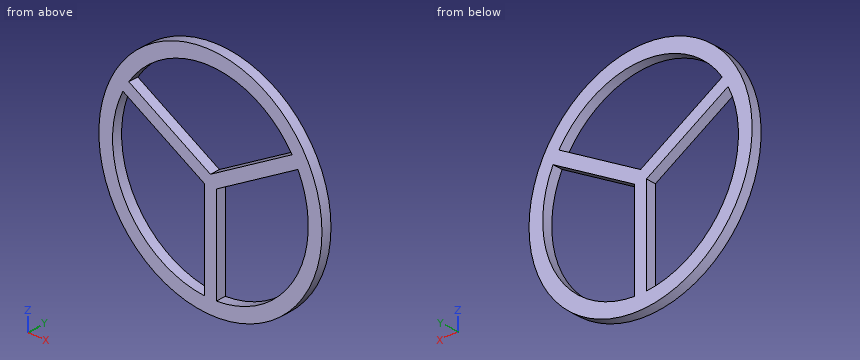
```python
from build123d import *

# Parameters (mm, degrees)
SKETCH1_R           = 28.5
SKETCH1_R_2         = 25
BOSS_EXTRUDE1_DEPTH = 2.5
BOSS_EXTRUDE2_DEPTH = 2.5


with BuildPart() as part:
    # Sketch1 → Boss-Extrude1 (new body)
    with BuildSketch(Plane(origin=(0, 0, 0), x_dir=(1, 0, 0), z_dir=(0, 1, 0))):
        Circle(SKETCH1_R)
        Circle(SKETCH1_R_2, mode=Mode.SUBTRACT)
    extrude(amount=BOSS_EXTRUDE1_DEPTH)

    # Sketch2 → Boss-Extrude2 (add)
    with BuildSketch(Plane(origin=(0, 2.5, 0), x_dir=(1, 0, 0), z_dir=(0, 1, 0))):
        Polygon((-1.5, 0.866025404), (-22.400635095, -11.200961894), (-20.900635095, -13.799038106), (0, -1.732050808), (20.900635095, -13.799038106), (22.400635095, -11.200961894), (1.5, 0.866025404), (1.5, 25), (-1.5, 25), align=None)
    extrude(amount=-BOSS_EXTRUDE2_DEPTH)


solid = part.part
```
Work out the finished part from the listing and answer in its coordinate system (mm). Round coordinates to 2 decimals unless told otherwise and drop trailing zeros. Write each loop counter-clockwise with the first axis right and the second up, starting at its lowest first coordinate (ties: lowest second). Pieces come first, ordered by that corner, then holes. Notation, with made-up numbers: (26, 62) -> (49, 62) arc R10 ccw to (49, 77) -> close; hole circle Ø6 at (83.25, -6.75). An arc over 180 degrees is marked (long way). Write each question's results on one line, items separated by ' | '.
1) The part is cut by section A-A (y = 1.3). Write down the section's boundary in (x, z), and give its area (3 significant figures).
Findings:
outline: circle Ø57 at (0, 0); hole (-22.36, 11.18) arc R25 ccw to (-1.5, -24.95) -> (-1.5, -0.87) -> close; hole (-20.86, 13.78) -> (0, 1.73) -> (20.86, 13.78) arc R25 ccw to start; hole (1.5, -24.95) arc R25 ccw to (22.36, 11.18) -> (1.5, -0.87) -> close | area: 809 mm²
2) The part is cut by section B-B (z = 0). Write down the section's boundary in (x, y).
Findings:
outline: (-28.5, 0) -> (-25, 0) -> (-25, 2.5) -> (-28.5, 2.5) -> close; (-3, 0) -> (3, 0) -> (3, 2.5) -> (-3, 2.5) -> close; (25, 0) -> (28.5, 0) -> (28.5, 2.5) -> (25, 2.5) -> close
3) Flat-ended cylindrical pins translate along their axes: pin 1 (2 mm diameter, centred on x = -20, z = 14.5, fed in from +Y); pin 2 (0.8 mm diameter, centred on y = 1, z = -11.5, fed in from -X); pin 3 (1 mm diameter, centred on x = 10.5, y = 1.5, fed in from -Z). Find the tip coordinate at first contact, or state that the pin passes through.
Findings:
pin 1: stops at y = 2.5 | pin 2: stops at x = -26.25 | pin 3: stops at z = -26.69
4) Consider line 1 along Z through (x, y) = (-2, 2); line 2 along X through (y, z) = (1.95, -5); line 3 along X through (y, z) = (1.2, -21.5). Determine where each line is inside the solid, lowest interval first. Write a range as [from, to].
Findings:
line 1: z = [-28.43, -24.92], [-0.58, 2.89], [24.92, 28.43] | line 2: x = [-28.06, -24.49], [-1.5, 1.5], [24.49, 28.06] | line 3: x = [-18.71, -12.76], [-1.5, 1.5], [12.76, 18.71]
5) The part is cut by section C-C (x = 9). Write down the section's boundary in (y, z).
Findings:
outline: (0, -27.04) -> (2.5, -27.04) -> (2.5, -23.32) -> (0, -23.32) -> close; (0, 3.46) -> (2.5, 3.46) -> (2.5, 6.93) -> (0, 6.93) -> close; (0, 23.32) -> (2.5, 23.32) -> (2.5, 27.04) -> (0, 27.04) -> close
